Design review of the part built by this model. Coordinates are the model's own, in mm. A direction names the side the tool comes from. Coordinates: 2 decimals unless noted, no trailing zeros. Loops run counter-clockwise (first coordinate to the right, second up) from the corner with the lowest first, then second, coordinate; pieces in that order, holes last. Notation, with made-up numbers: (25, -9) - (80, -9) arc R25 ccw to (80, 17) - close; hole circle Ø7 at (-11.75, 41). An arc over 180 degrees is marked (long way). One line per question, with ' | ' between items.
from build123d import *

# Parameters (mm, degrees)
SKETCH1_W             = 8.5
SKETCH1_H             = 8.5
EXTRUDE1_DEPTH        = 2.5
SKETCH15_W            = 7.7
SKETCH15_H            = 7.7
EXTRUDE8_DEPTH        = 0.5
SKETCH3_W             = 4
SKETCH3_H             = 2.5
EXTRUDE3_DEPTH        = 3.25
SKETCH2_W             = 7
SKETCH2_H             = 7
EXTRUDE2_DEPTH        = 1.5
EXTRUDE2_DEPTH_BACK   = 3.5
F_0_80_TAPPED_HOLE1_D = 1.19126
SKETCH11_W            = 2
SKETCH11_H            = 1
EXTRUDE5_DEPTH        = 1.5
FILLET1_R             = 1


with BuildPart() as part:
    # Sketch1 → Extrude1 (new body)
    with BuildSketch(Plane(origin=(0, 0, 0), x_dir=(1, 0, 0), z_dir=(0, 1, 0))):
        Rectangle(SKETCH1_W, SKETCH1_H)
    extrude(amount=EXTRUDE1_DEPTH)

    # Sketch15 → Extrude8 (add)
    with BuildSketch(Plane(origin=(0, 2.5, 0), x_dir=(1, 0, 0), z_dir=(0, 1, 0))):
        Rectangle(SKETCH15_W, SKETCH15_H)
    extrude(amount=EXTRUDE8_DEPTH)

    # Sketch3 → Extrude3 (add)
    with BuildSketch(Plane.XY.offset(4.25)):
        with Locations((-2.25, 1.25)):
            Rectangle(SKETCH3_W, SKETCH3_H)
    extrude(amount=EXTRUDE3_DEPTH)

    # Sketch2 → Extrude2 (cut, two sides)
    with BuildSketch(Plane(origin=(0, 2.5, 0), x_dir=(1, 0, 0), z_dir=(0, 1, 0))) as extrude2_sk:
        Rectangle(SKETCH2_W, SKETCH2_H)
    extrude(amount=EXTRUDE2_DEPTH, mode=Mode.SUBTRACT)
    extrude(extrude2_sk.sketch, amount=-EXTRUDE2_DEPTH_BACK, mode=Mode.SUBTRACT)

    # #0-80 Tapped Hole1 (through all)
    with Locations(Plane(origin=(-2.25, 2.5, 5.5), x_dir=(0, 0, 1), z_dir=(0, 1, 0))):
        with Locations((0, 0)):
            Hole(F_0_80_TAPPED_HOLE1_D / 2)

    # Sketch11 → Extrude5 (add)
    with BuildSketch(Plane(origin=(0, 0, -4.25), x_dir=(-1, 0, 0), z_dir=(0, 0, -1))):
        with Locations((-0.42960296, 0.5)):
            Rectangle(SKETCH11_W, SKETCH11_H)
    extrude(amount=EXTRUDE5_DEPTH)

    # Fillet1
    fillet1_edges = [part.edges().sort_by_distance(p)[0] for p in [
        (3.5, 1.5, -3.5),
        (-3.5, 1.5, -3.5),
        (-3.5, 1.5, 3.5),
        (3.5, 1.5, 3.5),
        (-4.25, 1.25, 7.5),
        (-0.25, 1.25, 7.5),
        (-0.25, 1.25, 4.25),
        (4.25, 1.25, 4.25),
        (4.25, 1.25, -4.25),
        (-4.25, 1.25, -4.25),
        (-3.85, 2.75, 3.85),
        (-3.85, 2.75, -3.85),
        (3.85, 2.75, -3.85),
        (3.85, 2.75, 3.85),
    ]]
    fillet(fillet1_edges, radius=FILLET1_R)


solid = part.part
Q1. For pin 1 (0.8 mm diameter, centred on x = 0.5, z = -5, fed in from +Y); pin 2 (0.6 mm diameter, centred on x = 1, y = 3, fed in from +Z); pin 3 (0.6 mm diameter, centred on x = -1.5, y = 2.5, fed in from -Z), all flat-tipped, find the tip position at first contact; note any pin that passes through.
Returned:
pin 1: stops at y = 1 | pin 2: stops at z = 3.85 | pin 3: stops at z = -4.25
Q2. Tool access review of faces 4 (the flat face through (3.5, 2, 0)), 5 (the flat face through (0, 1, -5)), 6 (the cylindrical face through (-3.565, 2.754, 3.549)), 7 (the cylindrical face through (-3.565, 2.754, -3.549)): name each direction out of +Z, -Z, +X, -X, +Y, -Y from which nothing blocks a thin tool from reaching the whole face with its end or side.
Returned:
face 4: +Y, -Y | face 5: -Z, +X, -X, +Y | face 6: +Z, -X, +Y | face 7: -Z, -X, +Y
Q3. Draft analysis for pull direction Z (two halves, no side actions). For faces 1 (the flat face through (-3.5, 2, 0)), 2 (the cylindrical face through (-3.965, 1.268, 7.199)), 3 (the flat face through (-0.57, 0.5, -5)), state which applies: +Z half, -Z half, draft (parallel to the pull), parting line (faces both ways), or undercut.
Returned:
face 1: undercut | face 2: +Z half | face 3: draft
Q4. Take a section at D-D (x = -0.75). Give the boundary of the cut face in (y, z).
Returned:
outline: (0, -4.25) - (2.5, -4.25) - (2.5, -3.85) - (3, -3.85) - (3, -3.5) - (0, -3.5) - close; (0, 3.5) - (3, 3.5) - (3, 3.85) - (2.5, 3.85) - (2.5, 7.37) - (0, 7.37) - close
Q5. Take a section at B-B (x = -2.25). Give the boundary of the cut face in (y, z), plus the area to 3 significant figures.
Returned:
outline: (0, -4.25) - (2.5, -4.25) - (2.5, -3.85) - (3, -3.85) - (3, -3.5) - (0, -3.5) - close; (0, 3.5) - (3, 3.5) - (3, 3.85) - (2.5, 3.85) - (2.5, 4.9) - (0, 4.9) - close; (0, 6.1) - (2.5, 6.1) - (2.5, 7.5) - (0, 7.5) - close | area: 9.25 mm²
Q6. Take a section at A-A (y = 1.55). Give the boundary of the cut face in (x, z).
Returned:
outline: (-4.25, -3.25) arc R1 ccw to (-3.25, -4.25) - (3.25, -4.25) arc R1 ccw to (4.25, -3.25) - (4.25, 3.25) arc R1 ccw to (3.25, 4.25) - (0.75, 4.25) arc R1 cw to (-0.25, 5.25) - (-0.25, 6.5) arc R1 ccw to (-1.25, 7.5) - (-3.25, 7.5) arc R1 ccw to (-4.25, 6.5) - close; hole (-3.5, -2.5) arc R1 ccw to (-2.5, -3.5) - (2.5, -3.5) arc R1 ccw to (3.5, -2.5) - (3.5, 2.5) arc R1 ccw to (2.5, 3.5) - (-2.5, 3.5) arc R1 ccw to (-3.5, 2.5) - close; hole circle Ø1.19 at (-2.25, 5.5)
Q7. To check wall thickness, follow line 1 along X through (y, z) = (2.1, -1); line 2 along X through (y, z) = (1.2, 5.5); line 3 along Z through (x, y) = (-1.75, 2.8). State the ranges of each line that lie inside material, in increasing order.
Returned:
line 1: x = -4.25 to -3.5, 3.5 to 4.25 | line 2: x = -4.25 to -2.85, -1.65 to -0.25 | line 3: z = -3.85 to -3.5, 3.5 to 3.85
Q8. Take a section at C-C (z = 5.5). Give the boundary of the cut face in (x, y), plus the area to 3 significant figures.
Returned:
outline: (-4.25, 0) - (-2.85, 0) - (-2.85, 2.5) - (-4.25, 2.5) - close; (-1.65, 0) - (-0.25, 0) - (-0.25, 2.5) - (-1.65, 2.5) - close | area: 7.02 mm²
